Build history of the part. All positions in model axes, mm. Face numbers are marked on the shaded views. A direction names the side the tool comes from. Give positions to 0.01 mm unless a question says otherwise; leave off trailing zeros. Loops run counter-clockwise (first coordinate to the right, second up) from the corner with the lowest first, then second, coordinate; pieces in that order, holes last. Notation, with made-up numbers: M 78.25,2.25 L 132.25,2.25 A17 cw 132.25,6.25 Z; hole C 3.5,-19 d9. An arc over 180 degrees is marked long. Answer in a Markdown table with one row per item. Add a question column.
```python
from build123d import *

# Parameters (mm, degrees)
SKETCH_1_R      = 2
EXTRUDE_1_DEPTH = 4
SKETCH_2_W      = 20
SKETCH_2_H      = 3
EXTRUDE_2_DEPTH = 10


with BuildPart() as part:
    # 草图1 → 凸台-拉伸1 (new body)
    with BuildSketch(Plane.XY):
        with BuildLine():
            Line((-10, -10), (10, -10))
            Line((10, -10), (3.512931993, 1.912931993))
            ThreePointArc((3.512931993, 1.912931993), (0, 4), (-3.512931993, 1.912931993))
            Line((-3.512931993, 1.912931993), (-10, -10))
        make_face()
        Circle(SKETCH_1_R, mode=Mode.SUBTRACT)
    extrude(amount=EXTRUDE_1_DEPTH)

    # 草图2 → 凸台-拉伸2 (add)
    with BuildSketch(Plane.XY.offset(4)):
        with Locations((0, -11.5)):
            Rectangle(SKETCH_2_W, SKETCH_2_H)
    extrude(amount=-EXTRUDE_2_DEPTH)


solid = part.part
```
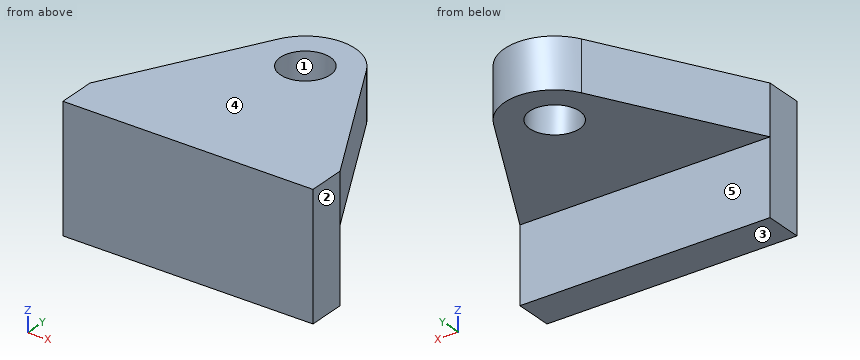
(1) Slice it at D-D, the plane z = -1.25. Give the cut face in (x, y), then the cut area to 3 significant figures.
(2) Slice it at B-B, the plane z = 2.5. Give the cut face in (x, y), then the cut area to 3 significant figures.
(3) Slice it at C-C, the plane y = 1.25. Give the cut face in (x, z), then the cut area to 3 significant figures.
(4) Slice it at A-A, the plane x = 0. Give the cut face in (y, z), then the cut area to 3 significant figures.
(5) Tool access for the marked faces 4 and 5: list every direction of +Z, -Z, +X, -X, +Y, -Y with a clear straight run to the whole face (end or side of a thin tool).
(6) Pin check, flat tips, straight feed: pin 1 (1.5 mm diameter, centred on x = -2, y = 2, fed in from -Z); pin 2 (4 mm diameter, centred on x = -8, z = 1, fed in from +Y); pin 3 (1.8 mm diameter, centred on x = 1, z = -3, fed in from +Y). Stop position of each tip, or through.
(7) Pull direction X, two halves, no side cores. Call the marked faces 1, 2 and 3: +X half, -X half, draft (parallel to the pull), parting line (faces both ways), or undercut.
(8) Wall check: line 1 (Z direction, x = 7.25, y = -6.25); line 2 (Y direction, x = 1, z = -2.25); line 3 (X direction, y = 0.75, z = 2.5). Give the ranges that are in metal, low to high.
Solution:
| question | item | result |
|---|---|---|
| 1 | outline | M -10,-13 L 10,-13 L 10,-10 L -10,-10 Z |
| 1 | area | 60.0 mm^2 |
| 2 | outline | M -10,-13 L 10,-13 L 10,-10 L 3.51,1.91 A4 ccw -3.51,1.91 L -10,-10 Z; hole C 0,0 d4 |
| 2 | area | 219 mm^2 |
| 3 | outline | M -3.87,0 L -1.56,0 L -1.56,4 L -3.87,4 Z; M 1.56,0 L 3.87,0 L 3.87,4 L 1.56,4 Z |
| 3 | area | 18.5 mm^2 |
| 4 | outline | M -13,-6 L -10,-6 L -10,0 L -2,0 L -2,4 L -13,4 Z; M 2,0 L 4,0 L 4,4 L 2,4 Z |
| 4 | area | 70.0 mm^2 |
| 5 | face 4 | +Z, +X, -X, +Y, -Y |
| 5 | face 5 | -Z, +X, -X, +Y |
| 6 | pin 1 | z = 0 |
| 6 | pin 2 | y = -2.65 |
| 6 | pin 3 | y = -10 |
| 7 | face 1 | undercut |
| 7 | face 2 | +X half |
| 7 | face 3 | draft |
| 8 | line 1 | 0 to 4 |
| 8 | line 2 | -13 to -10 |
| 8 | line 3 | -4.15 to -1.85, 1.85 to 4.15 |
